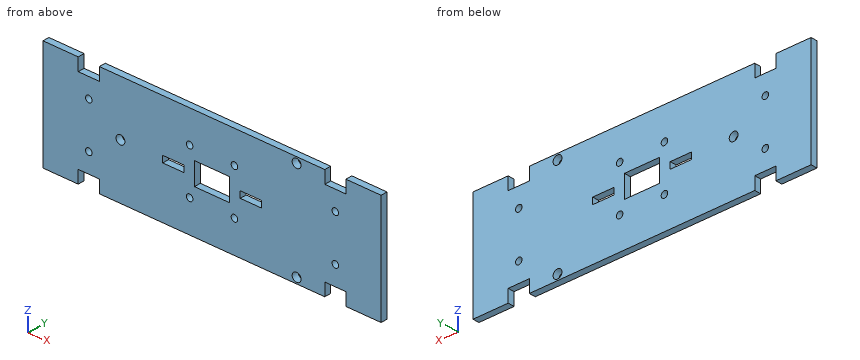
from build123d import *

# Parameters (mm, degrees)
SKETCH2_W                       = 9.525
SKETCH2_H                       = 2.9591
SKETCH2_W_2                     = 15.875
SKETCH2_H_2                     = 10.16
BOSS_EXTRUDE1_DEPTH             = 2.9591
F_4_CLEARANCE_HOLE1_D           = 2.9464
F_4_CLEARANCE_HOLE1_DEPTH       = 3.302
F_4_CLEARANCE_HOLE1_TIP         = 0.885187864
F_4_CLEARANCE_HOLE2_D           = 3.9624
F_4_CLEARANCE_HOLE2_DEPTH       = 3.302
F_4_CLEARANCE_HOLE2_TIP         = 1.190425058
TAP_DRILL_FOR_4_HELICOIL1_D     = 3.9878
TAP_DRILL_FOR_4_HELICOIL1_DEPTH = 5.588
TAP_DRILL_FOR_4_HELICOIL1_TIP   = 1.198055988


with BuildPart() as part:
    # Sketch2 → Boss-Extrude1 (new body)
    with BuildSketch(Plane(origin=(0, 0, 0), x_dir=(1, 0, 0), z_dir=(0, 1, 0))):
        Polygon((-76.2, 24.8158), (-60.325, 24.8158), (-60.325, 19.05), (-50.8, 19.05), (-50.8, 24.8158), (50.8, 24.8158), (50.8, 19.05), (60.325, 19.05), (60.325, 24.8158), (76.2, 24.8158), (76.2, -24.8158), (60.325, -24.8158), (60.325, -19.05), (50.8, -19.05), (50.8, -24.8158), (-50.8, -24.8158), (-50.8, -19.05), (-60.325, -19.05), (-60.325, -24.8158), (-76.2, -24.8158), align=None)
        with Locations((-17.4625, 0)):
            Rectangle(SKETCH2_W, SKETCH2_H, mode=Mode.SUBTRACT)
        with Locations((17.4625, 0)):
            Rectangle(SKETCH2_W, SKETCH2_H, mode=Mode.SUBTRACT)
        Rectangle(SKETCH2_W_2, SKETCH2_H_2, mode=Mode.SUBTRACT)
    extrude(amount=BOSS_EXTRUDE1_DEPTH)

    # #4 Clearance Hole1
    with Locations(Plane(origin=(0, 2.9591, 0), x_dir=(1, 0, 0), z_dir=(0, 1, 0))):
        with Locations((0, 0), (10.0965, 10.264775), (-10.0965, -10.264775), (-10.0965, 10.264775), (10.0965, -10.264775), (55.5625, 10.264775), (-55.5625, -10.264775), (55.5625, -10.264775), (-55.5625, 10.264775)):
            Hole(F_4_CLEARANCE_HOLE1_D / 2, depth=F_4_CLEARANCE_HOLE1_DEPTH)
            with Locations((0, 0, -(F_4_CLEARANCE_HOLE1_DEPTH + F_4_CLEARANCE_HOLE1_TIP / 2))):  # 118° drill point
                Cone(0, F_4_CLEARANCE_HOLE1_D / 2, F_4_CLEARANCE_HOLE1_TIP, mode=Mode.SUBTRACT)

    # #4 Clearance Hole2
    with Locations(Plane(origin=(0, 2.9591, 0), x_dir=(1, 0, 0), z_dir=(0, 1, 0))):
        with Locations((-41.275, 0)):
            Hole(F_4_CLEARANCE_HOLE2_D / 2, depth=F_4_CLEARANCE_HOLE2_DEPTH)
            with Locations((0, 0, -(F_4_CLEARANCE_HOLE2_DEPTH + F_4_CLEARANCE_HOLE2_TIP / 2))):  # 118° drill point
                Cone(0, F_4_CLEARANCE_HOLE2_D / 2, F_4_CLEARANCE_HOLE2_TIP, mode=Mode.SUBTRACT)

    # Tap Drill for #4 Helicoil1
    with Locations(Plane(origin=(0, 0, 0), x_dir=(-1, 0, 0), z_dir=(0, -1, 0))):
        with Locations((-38.1, 22.225), (-38.1, -22.225)):
            Hole(TAP_DRILL_FOR_4_HELICOIL1_D / 2, depth=TAP_DRILL_FOR_4_HELICOIL1_DEPTH)
            with Locations((0, 0, -(TAP_DRILL_FOR_4_HELICOIL1_DEPTH + TAP_DRILL_FOR_4_HELICOIL1_TIP / 2))):  # 118° drill point
                Cone(0, TAP_DRILL_FOR_4_HELICOIL1_D / 2, TAP_DRILL_FOR_4_HELICOIL1_TIP, mode=Mode.SUBTRACT)


solid = part.part
The listing builds one solid part. Answer for the finished solid, in the listing's coordinates (mm). Coordinates: 2 decimals unless noted, no trailing zeros. Loops run counter-clockwise (first coordinate to the right, second up) from the corner with the lowest first, then second, coordinate; pieces in that order, holes last.
1) Find section B-B on z = 0. Write down the section's boundary in (x, y) (1 decimal).
2) Find the intervals of material crossed by L1, parallel to Z at x = 38.1, y = 1.3; L2, parallel to X at y = 0.5, z = 4; L3, parallel to Z at x = -4.5, y = 2.3, in increasing order.
3) Find section A-A on x = 38.1. Write down the section's boundary in (y, z).
4) Find section C-C on y = 2.15. Give the number of separate pieces and of enclosed holes in the cut face, then the cut area to 3 significant figures.
5) Flat-ended cylindrical pins translate along their axes: pin 1 Ø0.9 at (x, y) = (-55.5, 2) entering from +Z; pin 2 Ø8 at (x, z) = (-37.5, 11.5) entering from -Y; pin 3 Ø1.5 at (x, y) = (-53.5, 2) entering from -Z. Find the tip coordinate at first contact, or state that the pin passes through.
Values:
1. outline: (-76.2, 0) - (-43.3, 0) - (-43.3, 3) - (-76.2, 3) - close; (-39.3, 0) - (-22.2, 0) - (-22.2, 3) - (-39.3, 3) - close; (-12.7, 0) - (-7.9, 0) - (-7.9, 3) - (-12.7, 3) - close; (7.9, 0) - (12.7, 0) - (12.7, 3) - (7.9, 3) - close; (22.2, 0) - (76.2, 0) - (76.2, 3) - (22.2, 3) - close
2. L1: z = -24.82 to -24.22, -20.23 to 20.23, 24.22 to 24.82
2. L2: x = -76.2 to -7.94, 7.94 to 76.2
2. L3: z = -24.82 to -5.08, 5.08 to 24.82
3. outline: (0, -24.82) - (2.96, -24.82) - (2.96, -24.22) - (0, -24.22) - close; (0, -20.23) - (2.96, -20.23) - (2.96, 20.23) - (0, 20.23) - close; (0, 24.22) - (2.96, 24.22) - (2.96, 24.82) - (0, 24.82) - close
4. separate pieces: 1
4. enclosed holes: 14
4. area: 7,030 mm2
5. pin 1: stops at z = 19.05
5. pin 2: stops at y = 0
5. pin 3: stops at z = -19.05
